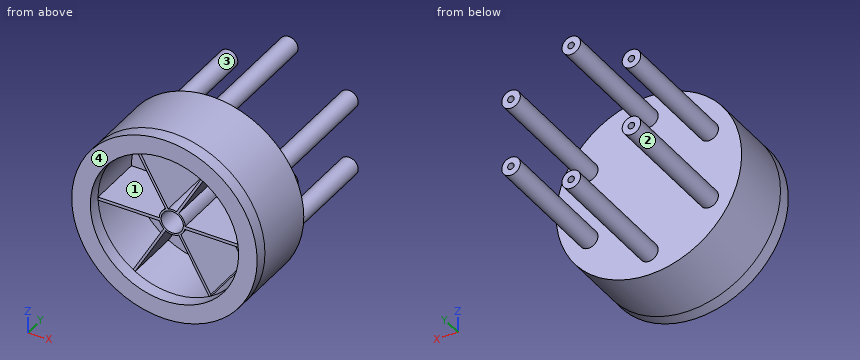
Autodesk Inventor part; units mm, degrees
ref_plane "YZ Plane" through (0, 0, 0) normal (1, 0, 0) x (0, 1, 0)
ref_plane "XZ Plane" through (0, 0, 0) normal (0, 1, 0) x (-1, 0, 0)
ref_plane "XY Plane" through (0, 0, 0) normal (0, 0, 1) x (1, 0, 0)
sketch "Boceto1" plane through (0, 0, 0) normal (0, 1, 0) x (-1, 0, 0)
  line L0 (0, 0) -> (100, 0) construction
  line L1 (100, 0) -> (100, 100) construction
  line L2 (100, 100) -> (0, 100) construction
  line L3 (0, 100) -> (0, 0) construction
  line L4 (0, 100) -> (100, 0) construction
  line L5 (100, 100) -> (0, 0) construction
  circle A0 centre (50, 50) radius 50
  dimension "d2" = 100
extrude "Extrusión1" add sketch "Boceto1" along normal blind 35
sketch "Boceto2" plane through (-50, 35, 50) normal (0, 1, 0) x (1, 0, 0)
  circle A0 centre (0, 0) radius 37.5 construction
  line L0 (0, 37.5) -> (32.476, 18.75) construction
  line L1 (32.476, 18.75) -> (32.476, -18.75) construction
  line L2 (32.476, -18.75) -> (0, -37.5) construction
  line L3 (0, -37.5) -> (-32.476, -18.75) construction
  line L4 (-32.476, -18.75) -> (-32.476, 18.75) construction
  line L5 (-32.476, 18.75) -> (0, 37.5) construction
  circle A1 centre (0, 37.5) radius 5
  circle A2 centre (32.476, 18.75) radius 5
  circle A3 centre (32.476, -18.75) radius 5
  circle A4 centre (0, -37.5) radius 5
  circle A5 centre (-32.476, -18.75) radius 5
  circle A6 centre (-32.476, 18.75) radius 5
  point P0 (50, 50)
  dimension "d5" = 75
  dimension "d6" = 10
  dimension "d7" = 10
  dimension "d8" = 10
  dimension "d9" = 10
  dimension "d10" = 10
  dimension "d11" = 10
extrude "Extrusión2" add sketch "Boceto2" along normal blind 70
sketch "Boceto3" plane through (-82.476, 105, 68.75) normal (0, 1, 0) x (1, 0, 0)
  circle A0 centre (32.5355, 18.7491) radius 37.5 construction
  circle A1 centre (32.5355, -18.7509) radius 1.75
  circle A2 centre (65.012, 0) radius 1.75
  circle A3 centre (65.012, 37.4981) radius 1.75
  circle A4 centre (32.5355, 56.2491) radius 1.75
  circle A5 centre (0.059, 37.4981) radius 1.75
  circle A6 centre (0, 0) radius 5
  circle A7 centre (0, 0) radius 1.75
  point P0 (82.476, 68.75)
  dimension "d15" = 3.5
  dimension "d16" = 3.5
  dimension "d17" = 3.5
  dimension "d18" = 3.5
  dimension "d19" = 3.5
  dimension "d20" = 3.5
extrude "Extrusión3" cut sketch "Boceto3" against normal blind 9 contours A1 | A2 | A3 | A4 | A5 | A7
sketch "Boceto4" plane through (-50, 0, 50) normal (0, -1, 0) x (1, 0, 0)
  circle A0 centre (0, 0) radius 40
  circle A1 centre (0, 0) radius 6
  line L0 (-20, -34.641) -> (-3.5, -6.0622)
  line L1 (-20.7581, -33.3279) -> (-4.5751, -5.298)
  line L2 (20, -34.641) -> (3.5, -6.0622)
  line L3 (-18.2769, 34.641) -> (-2.199, 6.6456)
  line L4 (4.6319, -5.2484) -> (20.7581, -33.3279)
  line L5 (39.0497, -1.6459) -> (6.8037, -1.6459)
  line L6 (7, 0) -> (40, 0)
  line L7 (3.5, 6.0622) -> (20, 34.641)
  line L8 (2.3007, 6.6111) -> (18.4837, 34.641)
  arc A2 (2.3007, 6.6111) -> (-2.199, 6.6456) centre (0, 0) ccw
  arc A3 (-3.5, 6.0622) -> (-7, 0) centre (0, 0) ccw
  line L9 (-6.8037, -1.6459) -> (-39.0497, -1.6459)
  arc A4 (-6.8037, -1.6459) -> (-4.5751, -5.298) centre (0, 0) ccw
  line L10 (-40, 0) -> (-7, 0)
  arc A5 (-3.5, -6.0622) -> (3.5, -6.0622) centre (0, 0) ccw
  arc A6 (4.6319, -5.2484) -> (6.8037, -1.6459) centre (0, 0) ccw
  arc A7 (7, 0) -> (3.5, 6.0622) centre (0, 0) ccw
  line L11 (-3.5, 6.0622) -> (-20, 34.641)
  line L12 (20.7581, -33.3279) -> (21.125, -33.9667)
  line L13 (39.0497, -1.6459) -> (39.9661, -1.6459)
  line L14 (18.4837, 34.641) -> (18.852, 35.2789)
  line L15 (-18.6921, 35.3639) -> (-18.2769, 34.641)
  line L16 (-39.0497, -1.6459) -> (-39.9661, -1.6459)
  line L17 (-20.7581, -33.3279) -> (-21.125, -33.9667)
  point P0 (50, -50)
  point P1 (-20, -34.641)
  point P2 (20, 34.641)
  point P3 (-20, 34.641)
  dimension "d23" = 80
  dimension "d24" = 12
extrude "Extrusión4" cut sketch "Boceto4" against normal blind 30 contours L6 A7 L7 A0 | A0 L12 L4 A6 L5 L13 | L14 L8 A2 L3 L15 A0 | A0 L0 A5 L2 | L11 A3 L10 A0 | A0 L16 L9 A4 L1 L17 | A1
sketch "Boceto5" plane through (-50, 0, 50) normal (0, -1, 0) x (1, 0, 0)
  arc A0 (-3.5, 6.0622) -> (-7, 0) centre (0, 0) ccw
  circle A1 centre (0, 0) radius 50
  circle A2 centre (0, 0) radius 40
  point P0 (50, -50)
  dimension "d28" = 100
  dimension "d29" = 80
extrude "Extrusión5" add sketch "Boceto5" along normal blind 7
thread "Rosca1"
The listing builds one solid part. Answer for the finished solid, in the listing's coordinates (mm). Face numbers are marked on the shaded views. A direction names the side the tool comes from. Coordinates: 2 decimals unless noted, no trailing zeros. Loops run counter-clockwise (first coordinate to the right, second up) from the corner with the lowest first, then second, coordinate; pieces in that order, holes last. Notation, with made-up numbers: M 68.5,7.5 L 94.5,7.5 A18 cw 94.5,16.5 Z; hole C -36,-39 d8. An arc over 180 degrees is marked long. Answer in a Markdown table with one row per item.
1) Which of the six approach directions +Z, -Z, +X, -X, +Y, -Y give full straight-line access (tool end or side, diameter ignored) to the marked faces 1 and 2?
Answers below:
| item | result |
|---|---|
| face 1 | -Y |
| face 2 | +Y |
2) Find the intervals of material crossed by probe 1 along Z at (x, y) = (-50, 10); probe 2 along X at (y, z) = (101, 68); probe 3 along X at (y, z) = (14.5, 62), in increasing order.
Answers below:
| item | result |
|---|---|
| probe 1 | 0 to 10, 43 to 44, 56 to 57, 90 to 100 |
| probe 2 | -87.42 to -84.06, -80.89 to -77.53, -22.47 to -19.05, -15.88 to -12.58 |
| probe 3 | -98.54 to -88.16, -56.93 to -55.27, -44.59 to -43.07, -11.84 to -1.46 |
3) Find section B-B (z = 60.5). Determine the outline of the cut face in (x, y).
Answers below:
| item | result |
|---|---|
| outline | M -98.89,-7 L -88.6,-7 L -88.6,30 L -56.06,30 L -56.06,0 L -54.41,0 L -54.41,30 L -45.45,30 L -45.45,0 L -43.94,0 L -43.94,30 L -11.4,30 L -11.4,-7 L -1.11,-7 L -1.11,35 L -98.89,35 Z |
4) Find section A-A (y = 80). Determine the outline of the cut face in (x, z), then the cut area to 3 significant figures.
Answers below:
| item | result |
|---|---|
| outline | C -82.48,31.25 d10; C -82.48,68.75 d10; C -50,12.5 d10; C -50,87.5 d10; C -17.52,31.25 d10; C -17.52,68.75 d10 |
| area | 471 mm^2 |
5) Given pin 1 (1.8 mm diameter, centred on x = -17.5, z = 69.5, fed in from +Y); pin 2 (4 mm diameter, centred on y = 36, z = 18.5, fed in from -X); pin 3 (10.5 mm diameter, centred on x = -28.5, z = 69.5, fed in from -Y), each flat-ended and moving along its own axis, determine where each tip first touches the part or whether it passes through.
Answers below:
| item | result |
|---|---|
| pin 1 | y = 96 |
| pin 2 | x = -90.17 |
| pin 3 | y = 30 |
6) Determine the mould class of the marked faces 3 and 4 for opening direction Z: released by +Z, released by -Z, zero draft, split by the parting line, or undercut.
Answers below:
| item | result |
|---|---|
| face 3 | undercut |
| face 4 | zero draft |
7) Find section C-C (y = 10). Count the separate pieces of the cut face and the enclosed holes in it, then the cut area to 3 significant figures.
Answers below:
| item | result |
|---|---|
| separate pieces | 1 |
| enclosed holes | 7 |
| area | 3,160 mm^2 |
